Read the model definition and answer for the solid it produces. Units are mm, in the model's axes. A direction names the side the tool comes from. Round coordinates to 2 decimals unless told otherwise and drop trailing zeros. Loops run counter-clockwise (first coordinate to the right, second up) from the corner with the lowest first, then second, coordinate; pieces in that order, holes last. Notation, with made-up numbers: (84.5, 5) - (135.5, 5) arc R23 ccw to (135.5, 25) - close; hole circle Ø1 at (26.5, 57). An arc over 180 degrees is marked (long way). Use CSV: the item, a comma, the result in double quotes. Start each with the question number.
1. Given pin 1 Ø7.5 at (x, y) = (-2.5, -2.5) entering from -Z; pin 2 Ø4 at (x, z) = (7, 13.5) entering from -Y; pin 3 Ø4 at (x, y) = (0, 0) entering from +Z; pin 4 Ø1.5 at (x, z) = (2, 13.5) entering from +Y, each flat-ended and moving along its own axis, determine where each tip first touches the part or whether it passes through.
2. Find section B-B (x = 0). Give the vertices of the cut face in (y, z) (3 decimals).
3. A tool of negligible diameter and unlimited length cuts with its end or side. For faces 1 (the flat face through (-5, -5, 34.6)), 2 (the flat face through (6.3, -1.6, 31.4)), 3 (the cylindrical face through (1.07, 8.13, 17.25)), from which of +Z, -Z, +X, -X, +Y, -Y can it reach the whole face along a straight path? Write none if from no direction.
4. Consider line 1 along Y through (x, z) = (0, 17.75); line 2 along Y through (x, z) = (0, 27.7) (3 decimals); line 3 along Z through (x, y) = (4, -14). Determine where each line is inside the solid, lowest interval first.
5. Find section C-C (x = 6). Give the vertices of the cut face in (y, z).
6. Find section A-A (y = 0). Give the vertices of the cut face in (x, z) (3 decimals).
7. Determine the mould class of faces 4 (the flat face through (-6.3, 1.6, 31.4)), 5 (the cylindrical face through (2.994, 22.804, 32.921)), 6 (the flat face through (-1.775, 6.253, 31.396)), 7 (the flat face through (11, 5, 31.289)) for opening direction Y: +Y half, -Y half, draft (parallel to the pull), parting line (faces both ways), or undercut.
8. Find section D-D (z = 13.5). Give the vertices of the cut face in (x, y), and give its area (3 significant figures).
from build123d import *

# Parameters (mm, degrees)
F0_W     = 0.7
F0_H     = 7.9574310766
F2_R     = 3.525
F3_DEPTH = 6.5


# Not quite as in the source:
# - a feature names something its author has since deleted; it is built from what else it names


with BuildPart() as f1:
    # F0 (on Front) → F1 (revolve)
    with BuildSketch(Plane.XZ):
        Polygon((-8.2, 24.3467036635), (-8.2, 18.3), (-7.5, 18.3), (-7.5, 20.7), (-7.5, 27), (-3.525, 27), (-3.525, 28.3), (-3.525, 34.6), (-23, 34.6), (-23, 31.2892384827), (-11.8090426549, 31.2892384827), (-11.8090426549, 26.945874095), (-11.8090426549, 24.3467036635), align=None)
        with Locations((-7.85, 14.3212844617)):
            Rectangle(F0_W, F0_H)
    revolve(axis=Axis((0, 0, 19.15), (0, 0, -1)))

    # F2 (on face) → F3 (cut)
    with BuildSketch(Plane.XY.offset(34.6)):
        Polygon((-7.2035379805, -2.107693976), (-1.7764524637, -7.2922938762), (5.4270855169, -5.1845999003), (7.2035379805, 2.107693976), (1.7764524637, 7.2922938762), (-5.4270855169, 5.1845999003), align=None)
        Circle(F2_R, mode=Mode.SUBTRACT)
    extrude(amount=-F3_DEPTH, mode=Mode.SUBTRACT)


solid = f1.part
Filled sheet:
1,pin 1,"stops at z = 27"
1,pin 2,"stops at y = -6.5"
1,pin 3,"passes through"
1,pin 4,"stops at y = 8.1"
2,outline,"(-23, 31.289) - (-11.809, 31.289) - (-11.809, 24.347) - (-8.2, 24.347) - (-8.2, 10.343) - (-7.5, 10.343) - (-7.5, 27) - (-3.525, 27) - (-3.525, 28.1) - (-6.773, 28.1) - (-6.773, 34.6) - (-23, 34.6) - close; (3.525, 27) - (7.5, 27) - (7.5, 10.343) - (8.2, 10.343) - (8.2, 24.347) - (11.809, 24.347) - (11.809, 31.289) - (23, 31.289) - (23, 34.6) - (6.773, 34.6) - (6.773, 28.1) - (3.525, 28.1) - close"
3,face 1,"+Z, +X, -X, +Y, -Y"
3,face 2,"+Z"
3,face 3,"-Z"
4,line 1,"y = -8.2 to -7.5, 7.5 to 8.2"
4,line 2,"y = -11.809 to -3.525, 3.525 to 11.809"
4,line 3,"z = 31.29 to 34.6"
5,outline,"(-22.2, 31.29) - (-10.17, 31.29) - (-10.17, 24.35) - (-5.59, 24.35) - (-5.59, 10.34) - (-4.5, 10.34) - (-4.5, 27) - (4.5, 27) - (4.5, 10.34) - (5.59, 10.34) - (5.59, 24.35) - (10.17, 24.35) - (10.17, 31.29) - (22.2, 31.29) - (22.2, 34.6) - (3.26, 34.6) - (3.26, 28.1) - (-2.83, 28.1) - (-2.83, 34.6) - (-22.2, 34.6) - close"
6,outline,"(-23, 31.289) - (-11.809, 31.289) - (-11.809, 24.347) - (-8.2, 24.347) - (-8.2, 10.343) - (-7.5, 10.343) - (-7.5, 27) - (-3.525, 27) - (-3.525, 28.1) - (-6.69, 28.1) - (-6.69, 34.6) - (-23, 34.6) - close; (3.525, 27) - (7.5, 27) - (7.5, 10.343) - (8.2, 10.343) - (8.2, 24.347) - (11.809, 24.347) - (11.809, 31.289) - (23, 31.289) - (23, 34.6) - (6.69, 34.6) - (6.69, 28.1) - (3.525, 28.1) - close"
7,face 4,"undercut"
7,face 5,"parting line"
7,face 6,"undercut"
7,face 7,"draft"
8,outline,"circle Ø16.4 at (0, 0); hole circle Ø15 at (0, 0)"
8,area,"34.5 mm²"
